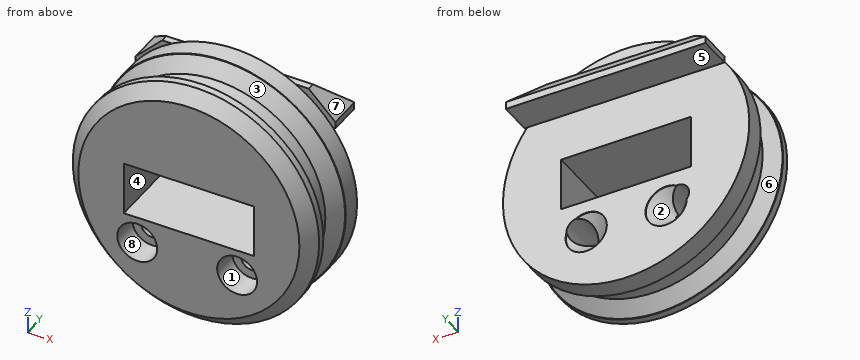
```python
from build123d import *

# Parameters (mm, degrees)
CYLINDER027_R             = 3
CYLINDER027_DEPTH         = 4
BOX005009016_W            = 16
BOX005009016_H            = 5.6
BOX005009016_DEPTH        = 3
CYLINDER026_R             = 1.7
CYLINDER026_DEPTH         = 30
FUSION026_PITCH_ANGLE     = 90
FUSION026_PLACEMENT_ANGLE = 90
FUSION025_PITCH_ANGLE     = 90
FUSION025_PLACEMENT_ANGLE = 90
BOX005009013_W            = 19.5
BOX005009013_H            = 400
BOX005009013_DEPTH        = 8
CYLINDER023_R             = 3.1
CYLINDER023_DEPTH         = 6
CYLINDER023_ROLL_ANGLE    = 90
CHAMFER015_SIZE           = 2.9
CHAMFER013_SIZE           = 2.9
CYLINDER021_R             = 18.5
CYLINDER021_DEPTH         = 3
CYLINDER021_ROLL_ANGLE    = 90
CYLINDER020_R             = 16.5
CYLINDER020_DEPTH         = 10
CYLINDER020_ROLL_ANGLE    = 90
CYLINDER019_R             = 18.5
CYLINDER019_DEPTH         = 3
CYLINDER019_ROLL_ANGLE    = 90
BOX005009014_W            = 30
BOX005009014_H            = 5
BOX005009014_DEPTH        = 5
CHAMFER016_SIZE           = 4
CHAMFER017_SIZE           = 4
CHAMFER018_SIZE           = 3.9
CHAMFER020_SIZE           = 1.9
CHAMFER021_SIZE           = 1.9
CHAMFER022_SIZE           = 1.9


with BuildPart() as cylinder018:
    # Cylinder027 → Cylinder027 (new body)
    with BuildSketch(Plane.XY):
        Circle(CYLINDER027_R)
    extrude(amount=CYLINDER027_DEPTH)


with BuildPart() as cube003:
    # Box005009016 → Box005009016 (new body)
    with BuildSketch(Plane(origin=(-3.2, -2.8, 18), x_dir=(1, 0, 0), z_dir=(0, 0, 1))):
        with Locations((8, 2.8)):
            Rectangle(BOX005009016_W, BOX005009016_H)
    extrude(amount=BOX005009016_DEPTH)


with BuildPart() as cylinder017:
    # Cylinder026 → Cylinder026 (new body)
    with BuildSketch(Plane.XY.offset(1)):
        Circle(CYLINDER026_R)
    extrude(amount=CYLINDER026_DEPTH)


with BuildPart() as m3_cavity003:
    # Fusion026 base: copy of Cylinder017
    add(cylinder017.part)

    # Fusion026: union Cylinder018, Cube003
    add(cylinder018.part)
    add(cube003.part)


with BuildPart() as m3_cavity003_1:
    # Fusion026 pitch: moved
    add(m3_cavity003.part.rotate(Axis((0, 0, 0), (0, 1, 0)), FUSION026_PITCH_ANGLE))


with BuildPart() as m3_cavity003_2:
    # Fusion026 placement: moved
    add(m3_cavity003_1.part.moved(Location((15, 249, -6))).rotate(Axis((15, 249, -6), (0, 0, 1)), FUSION026_PLACEMENT_ANGLE))


with BuildPart() as m3_cavity002:
    # Fusion025 base: copy of Cylinder017
    add(cylinder017.part)

    # Fusion025: union Cylinder018, Cube003
    add(cylinder018.part)
    add(cube003.part)


with BuildPart() as m3_cavity002_1:
    # Fusion025 pitch: moved
    add(m3_cavity002.part.rotate(Axis((0, 0, 0), (0, 1, 0)), FUSION025_PITCH_ANGLE))


with BuildPart() as m3_cavity002_2:
    # Fusion025 placement: moved
    add(m3_cavity002_1.part.moved(Location((0, 249, -6))).rotate(Axis((0, 249, -6), (0, 0, 1)), FUSION025_PLACEMENT_ANGLE))


with BuildPart() as scale_hole002:
    # Box005009013 → Box005009013 (new body)
    with BuildSketch(Plane(origin=(-2, 0, -2), x_dir=(1, 0, 0), z_dir=(0, 0, 1))):
        with Locations((9.75, 200)):
            Rectangle(BOX005009013_W, BOX005009013_H)
    extrude(amount=BOX005009013_DEPTH)


with BuildPart() as lug_hole:
    # Cylinder023 → Cylinder023 (new body)
    with BuildSketch(Plane.XY):
        Circle(CYLINDER023_R)
    extrude(amount=CYLINDER023_DEPTH)


with BuildPart() as lug_hole_1:
    # Cylinder023 roll: moved
    add(lug_hole.part.rotate(Axis((0, 0, 0), (1, 0, 0)), CYLINDER023_ROLL_ANGLE))


with BuildPart() as lug_hole_2:
    # Cylinder023 placement: moved
    add(lug_hole_1.part.moved(Location((7.75, 328, -7))))


with BuildPart() as chamfer015:
    # Chamfer015 base: copy of lug-hole
    add(lug_hole_2.part)

    # Chamfer015
    chamfer015_edges = [chamfer015.edges().sort_by_distance(p)[0] for p in [
        (4.65, 328, -7),
    ]]
    chamfer(chamfer015_edges, length=CHAMFER015_SIZE)


with BuildPart() as chamfer015_1:
    # Chamfer015 placement: moved
    add(chamfer015.part.moved(Location((6, 0, 0))))


with BuildPart() as part_mirroring003:
    # Part__Mirroring003: instance of Chamfer015
    add(chamfer015_1.part.mirror(Plane(origin=(0, 200, 0), x_dir=(1, 0, 0), z_dir=(0, 1, 0))))


with BuildPart() as chamfer013:
    # Chamfer013 base: copy of lug-hole
    add(lug_hole_2.part)

    # Chamfer013
    chamfer013_edges = [chamfer013.edges().sort_by_distance(p)[0] for p in [
        (4.65, 328, -7),
    ]]
    chamfer(chamfer013_edges, length=CHAMFER013_SIZE)


with BuildPart() as chamfer013_1:
    # Chamfer013 placement: moved
    add(chamfer013.part.moved(Location((-6, 0, 0))))


with BuildPart() as fusion017:
    # Part__Mirroring001: instance of Chamfer013
    add(chamfer013_1.part.mirror(Plane(origin=(0, 200, 0), x_dir=(1, 0, 0), z_dir=(0, 1, 0))))

    # Fusion017: union Part__Mirroring003
    add(part_mirroring003.part)


with BuildPart() as fusion017_1:
    # Fusion017 placement: moved
    add(fusion017.part.moved(Location((0, 186, 0))))


with BuildPart() as end_cheek002:
    # Cylinder021 → Cylinder021 (new body)
    with BuildSketch(Plane.XY):
        Circle(CYLINDER021_R)
    extrude(amount=CYLINDER021_DEPTH)


with BuildPart() as end_cheek002_1:
    # Cylinder021 roll: moved
    add(end_cheek002.part.rotate(Axis((0, 0, 0), (1, 0, 0)), CYLINDER021_ROLL_ANGLE))


with BuildPart() as end_cheek002_2:
    # Cylinder021 placement: moved
    add(end_cheek002_1.part.moved(Location((7.75, 486, 2))))


with BuildPart() as cable_tie_cyl002:
    # Cylinder020 → Cylinder020 (new body)
    with BuildSketch(Plane.XY):
        Circle(CYLINDER020_R)
    extrude(amount=CYLINDER020_DEPTH)


with BuildPart() as cable_tie_cyl002_1:
    # Cylinder020 roll: moved
    add(cable_tie_cyl002.part.rotate(Axis((0, 0, 0), (1, 0, 0)), CYLINDER020_ROLL_ANGLE))


with BuildPart() as cable_tie_cyl002_2:
    # Cylinder020 placement: moved
    add(cable_tie_cyl002_1.part.moved(Location((7.75, 485, 2))))


with BuildPart() as cut020:
    # Cylinder019 → Cylinder019 (new body)
    with BuildSketch(Plane.XY):
        Circle(CYLINDER019_R)
    extrude(amount=CYLINDER019_DEPTH)


with BuildPart() as cut020_1:
    # Cylinder019 roll: moved
    add(cut020.part.rotate(Axis((0, 0, 0), (1, 0, 0)), CYLINDER019_ROLL_ANGLE))


with BuildPart() as cut020_2:
    # Cylinder019 placement: moved
    add(cut020_1.part.moved(Location((7.75, 477, 2))))

    # Fusion012: union end-cheek002, cable-tie-cyl002
    add(end_cheek002_2.part)
    add(cable_tie_cyl002_2.part)


with BuildPart() as cut020_3:
    # Fusion012 placement: moved
    add(cut020_2.part.moved(Location((0, -225, 0))))

    # Cut017: cut Fusion017
    add(fusion017_1.part, mode=Mode.SUBTRACT)

    # Cut020: cut scale-hole002
    add(scale_hole002.part, mode=Mode.SUBTRACT)


with BuildPart() as slide_end_r:
    # Box005009014 → Box005009014 (new body)
    with BuildSketch(Plane(origin=(-7, 261, 13), x_dir=(1, 0, 0), z_dir=(0, 0, 1))):
        with Locations((15, 2.5)):
            Rectangle(BOX005009014_W, BOX005009014_H)
    extrude(amount=BOX005009014_DEPTH)

    # Chamfer016
    chamfer016_edges = [slide_end_r.edges().sort_by_distance(p)[0] for p in [
        (-7, 263.5, 18),
    ]]
    chamfer(chamfer016_edges, length=CHAMFER016_SIZE)

    # Chamfer017
    chamfer017_edges = [slide_end_r.edges().sort_by_distance(p)[0] for p in [
        (23, 263.5, 18),
    ]]
    chamfer(chamfer017_edges, length=CHAMFER017_SIZE)

    # Chamfer018
    chamfer018_edges = [slide_end_r.edges().sort_by_distance(p)[0] for p in [
        (8, 266, 18),
    ]]
    chamfer(chamfer018_edges, length=CHAMFER018_SIZE)

    # Fusion020: union Cut020
    add(cut020_3.part)

    # Chamfer020
    chamfer020_edges = [slide_end_r.edges().sort_by_distance(p)[0] for p in [
        (-8.75, 252, 2),
    ]]
    chamfer(chamfer020_edges, length=CHAMFER020_SIZE)

    # Chamfer021
    chamfer021_edges = [slide_end_r.edges().sort_by_distance(p)[0] for p in [
        (-10.75, 249, 2),
    ]]
    chamfer(chamfer021_edges, length=CHAMFER021_SIZE)

    # Chamfer022
    chamfer022_edges = [slide_end_r.edges().sort_by_distance(p)[0] for p in [
        (-8.75, 258, 2),
    ]]
    chamfer(chamfer022_edges, length=CHAMFER022_SIZE)

    # Cut025: cut M3-cavity002
    add(m3_cavity002_2.part, mode=Mode.SUBTRACT)

    # Cut026: cut M3-cavity003
    add(m3_cavity003_2.part, mode=Mode.SUBTRACT)


solid = slide_end_r.part
```
Input: part model. Units: mm. Frame: model coordinates. Face numbers are marked on the shaded views. A direction names the side the tool comes from. Give positions to 0.01 mm unless a question says otherwise; leave off trailing zeros. Loops run counter-clockwise (first coordinate to the right, second up) from the corner with the lowest first, then second, coordinate; pieces in that order, holes last. Notation, with made-up numbers: M 31,-15.75 L 59,-15.75 A20 ccw 59,23.25 Z; hole C 54.5,-36 d2. An arc over 180 degrees is marked long. Answer as CSV lines item,"result". Start each with the question number.
1. Section A-A on x = 7.75. Return loops of the section in (y, z), plus the area to 3 significant figures.
2. Line query: L1, parallel to Z at x = 16.5, y = 254; L2, parallel to Z at x = -0.5, y = 252.25; L3, parallel to X at y = 260.75, z = 5.5. Output: solid intervals per line, ascending.
3. Pin query (flat end, axial travel): P1, Ø8, axis at y = 263, z = 7, coming from the +X side; P2, Ø3.5, axis at x = 6, y = 255.5, coming from the -Z side; P3, Ø7, axis at x = 1.75, z = -7, coming from the +Y side; P4, Ø3, axis at y = 263, z = -7.5, coming from the -X side. Return the tip coordinate at first contact, or that it passes through.
4. Section B-B on y = 251.5. Return loops of the section in (x, z).
5. Section C-C on y = 254.75. Return loops of the section in (x, z), plus the area to 3 significant figures.
6. Pull-direction query (Y, two-part tool) for the marked faces 1, 2 and 3; classes: released by +Y, released by -Y, zero draft, split by the parting line, or undercut.
7. Reachability of the marked faces 4, 5, 6, 7 and 8 from +Z, -Z, +X, -X, +Y, -Y: full face, straight path, thin tool, end or side. Return the list, or none.
Computed values:
1,outline,"M 249,-14.6 L 250.9,-16.5 L 252,-16.5 L 252,-16.4 L 253.9,-14.5 L 256.1,-14.5 L 258,-16.4 L 258,-16.5 L 261,-16.5 L 261,-2 L 249,-2 Z; M 249,6 L 261,6 L 261,13 L 266,13 L 266,14.1 L 262.1,18 L 261,18 L 261,20.5 L 258,20.5 L 258,20.4 L 256.1,18.5 L 253.9,18.5 L 252,20.4 L 252,20.5 L 250.9,20.5 L 249,18.6 Z"
1,area,"345 mm²"
2,L1,"z = -11.99 to -6.8, -5.2 to -2, 6 to 15.99"
2,L2,"z = -14.17 to -8.96, -3.04 to -2, 6 to 18.17"
2,L3,"x = -10.42 to -2, 17.5 to 25.92"
3,P1,"stops at x = 26.19"
3,P2,"stops at z = -15.57"
3,P3,"stops at y = 261"
3,P4,"passes through"
4,outline,"C 7.75,2 d37; hole C 0,-6 d6; hole M -2,-2 L 17.5,-2 L 17.5,6 L -2,6 Z; hole C 15,-6 d6"
5,outline,"C 7.75,2 d33; hole M -2,-2 L 17.5,-2 L 17.5,6 L -2,6 Z; hole C 0,-6 d3.4; hole C 15,-6 d3.4"
5,area,"681 mm²"
6,face 1,"zero draft"
6,face 2,"released by +Y"
6,face 3,"undercut"
7,face 4,"+Y, -Y"
7,face 5,"-Z, +X, -X, +Y"
7,face 6,"none"
7,face 7,"+Z, +X, +Y, -Y"
7,face 8,"-Y"
